Could you check a few things on this drawing? It's one solid part, dimensions in mm from its lowest x, y, z. Coordinates: 2 decimals unless noted, no trailing zeros. Loops run counter-clockwise (first coordinate to the right, second up) from the corner with the lowest first, then second, coordinate; pieces in that order, holes last.
1) Imagine slicing it at B-B on z = 18. Please give me the cut outline in (x, y) (1 decimal).
2) Thinking about a two-plate mould opening in Z: for the marked faces 1 and 2, which applies, released by +Z, released by -Z, zero draft, split by the parting line, or undercut?
3) Imagine slicing it at C-C on y = 2.75. Please give me the cut outline in (x, z) (1 decimal).
4) Will these pins go through, and if not, where does the flat tip stop? P1, Ø5, axis at x = 79.51, z = 58.17, coming from the +Y side (1 decimal); P2, Ø4, axis at x = 73.09, z = 67.5, coming from the -Y side; P3, Ø2.5, axis at x = 48, y = 6.5, coming from the +Z side; P4, Ø2.5, axis at x = 12.5, y = 6.5, coming from the +Z side.
5) Imagine slicing it at D-D on z = 49.5. Please give me the cut outline in (x, y) (1 decimal).
6) If I drill on line 1 along X through (y, z) = (6.25, 34) (1 decimal); line 2 along X through (y, z) = (6.75, 67.5) (1 decimal); line 3 along X through (y, z) = (0.5, 11.5), over which ranges is the centre line in solid material (lowest first)?
7) Imagine slicing it at A-A on z = 34. Please give me the cut outline in (x, y) (1 decimal), plus the area to 3 significant figures.
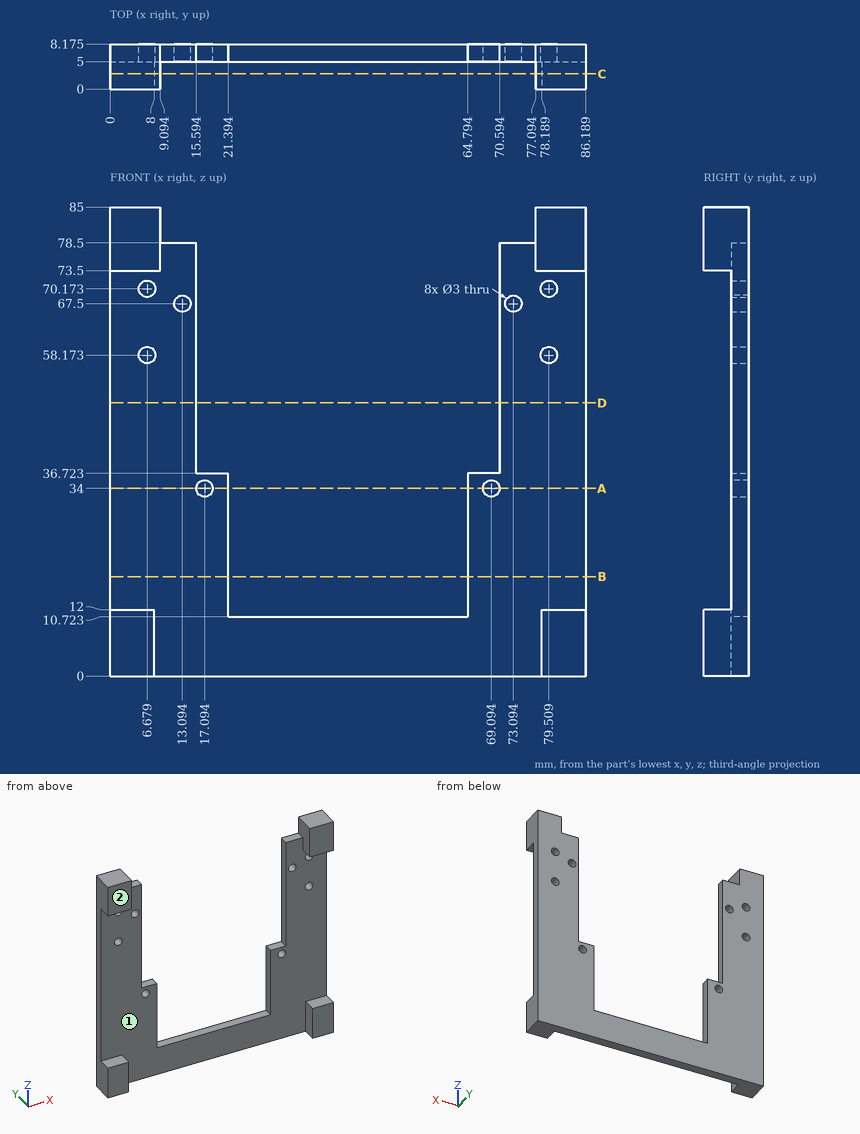
Filled in:
1. outline: (0, 5) - (21.4, 5) - (21.4, 8.2) - (0, 8.2) - close; (64.8, 5) - (86.2, 5) - (86.2, 8.2) - (64.8, 8.2) - close
2. face 1: undercut
2. face 2: zero draft
3. outline: (0, 0) - (8, 0) - (8, 12) - (0, 12) - close; (0, 73.5) - (9.1, 73.5) - (9.1, 85) - (0, 85) - close; (77.1, 73.5) - (86.2, 73.5) - (86.2, 85) - (77.1, 85) - close; (78.2, 0) - (86.2, 0) - (86.2, 12) - (78.2, 12) - close
4. P1: stops at y = 8.2
4. P2: stops at y = 5
4. P3: stops at z = 10.72
4. P4: stops at z = 78.5
5. outline: (0, 5) - (15.6, 5) - (15.6, 8.2) - (0, 8.2) - close; (70.6, 5) - (86.2, 5) - (86.2, 8.2) - (70.6, 8.2) - close
6. line 1: x = 0 to 15.6, 18.6 to 21.4, 64.8 to 67.6, 70.6 to 86.2
6. line 2: x = 0 to 11.6, 14.6 to 15.6, 70.6 to 71.6, 74.6 to 86.2
6. line 3: x = 0 to 8, 78.19 to 86.19
7. outline: (0, 5) - (15.6, 5) - (15.6, 8.2) - (0, 8.2) - close; (18.6, 5) - (21.4, 5) - (21.4, 8.2) - (18.6, 8.2) - close; (64.8, 5) - (67.6, 5) - (67.6, 8.2) - (64.8, 8.2) - close; (70.6, 5) - (86.2, 5) - (86.2, 8.2) - (70.6, 8.2) - close
7. area: 117 mm2
